The model under review builds one solid part; all positions refer to its coordinate system, in mm. Give positions to 0.01 mm unless a question says otherwise; leave off trailing zeros. Loops run counter-clockwise (first coordinate to the right, second up) from the corner with the lowest first, then second, coordinate; pieces in that order, holes last. Notation, with made-up numbers: M 25,63 L 46,63 A28 ccw 46,81 Z; hole C 15.5,25 d2. An arc over 180 degrees is marked long. Return JSON: item names as keys, results as strings. Group by question number.
```python
from build123d import *

# Parameters (mm, degrees)
SKETCH_1_W      = 220
SKETCH_1_H      = 54
SKETCH_1_R      = 2.1
SKETCH_1_R_2    = 2
SKETCH_1_R_3    = 14.5
EXTRUDE_1_DEPTH = 3
CHAMFER_1_SIZE  = 4


with BuildPart() as part:
    # 草图1 → 凸台-拉伸1 (new, symmetric)
    with BuildSketch(Plane.XY):
        Rectangle(SKETCH_1_W, SKETCH_1_H)
        with Locations((-100, 17)):
            Circle(SKETCH_1_R, mode=Mode.SUBTRACT)
        with Locations((-100, -17)):
            Circle(SKETCH_1_R, mode=Mode.SUBTRACT)
        with Locations((100, 17)):
            Circle(SKETCH_1_R, mode=Mode.SUBTRACT)
        with Locations((100, -17)):
            Circle(SKETCH_1_R, mode=Mode.SUBTRACT)
        with Locations((0, 17.5)):
            Circle(SKETCH_1_R_2, mode=Mode.SUBTRACT)
        Circle(SKETCH_1_R_3, mode=Mode.SUBTRACT)
        with Locations((17.5, 0)):
            Circle(SKETCH_1_R_2, mode=Mode.SUBTRACT)
        with Locations((0, -17.5)):
            Circle(SKETCH_1_R_2, mode=Mode.SUBTRACT)
        with Locations((-17.5, 0)):
            Circle(SKETCH_1_R_2, mode=Mode.SUBTRACT)
    extrude(amount=EXTRUDE_1_DEPTH, both=True)

    # 倒角1
    chamfer_1_edges = [part.edges().sort_by_distance(p)[0] for p in [
        (-110, 27, 0),
        (110, 27, 0),
        (110, -27, 0),
        (-110, -27, 0),
    ]]
    chamfer(chamfer_1_edges, length=CHAMFER_1_SIZE)


solid = part.part
```
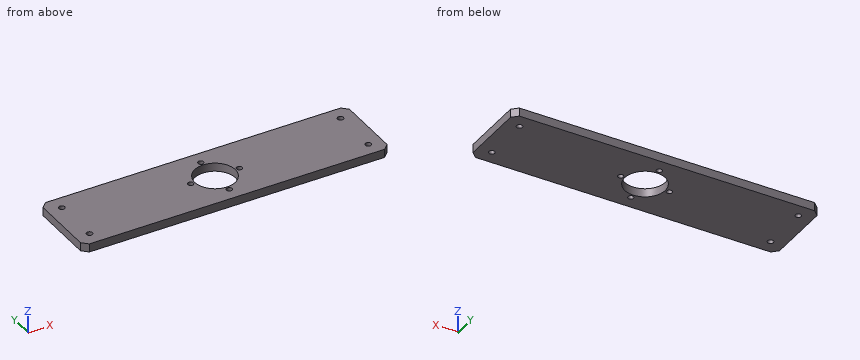
(1) For probe 1 along Y at (x, z) = (0, -1.7); probe 2 along Y at (x, z) = (100, 0.9); probe 3 along Y at (x, z) = (17.5, 0), list the stretches that pass through material, from the lowest coordinate up.
(2) Add section B-B (x = -100). Write out the cut boundary in (y, z), and give its area (3 significant figures).
(3) Add section C-C (y = -10). Write out the cut boundary in (x, z), and give its area (3 significant figures).
(4) Add section D-D (x = 6). Write out the cut boundary in (y, z).
(5) For pin 1 (6.5 mm diameter, centred on x = 17.5, y = 0, fed in from -Z), flat-tipped, find the tip position at first contact; note if it passes through.
(6) Add section A-A (z = 1.25). Count the separate pieces of the cut face and the enclosed holes in it, and give its area (3 significant figures).
Verdict:
{
 "1": {"probe 1": "y = -27 to -19.5, -15.5 to -14.5, 14.5 to 15.5, 19.5 to 27", "probe 2": "y = -27 to -19.1, -14.9 to 14.9, 19.1 to 27", "probe 3": "y = -27 to -2, 2 to 27"},
 "2": {"outline": "M -27,-3 L -19.1,-3 L -19.1,3 L -27,3 Z; M -14.9,-3 L 14.9,-3 L 14.9,3 L -14.9,3 Z; M 19.1,-3 L 27,-3 L 27,3 L 19.1,3 Z", "area": "274 mm²"},
 "3": {"outline": "M -110,-3 L -10.5,-3 L -10.5,3 L -110,3 Z; M 10.5,-3 L 110,-3 L 110,3 L 10.5,3 Z", "area": "1,190 mm²"},
 "4": {"outline": "M -27,-3 L -13.2,-3 L -13.2,3 L -27,3 Z; M 13.2,-3 L 27,-3 L 27,3 L 13.2,3 Z"},
 "5": {"pin 1": "stops at z = -3"},
 "6": {"separate pieces": "1", "enclosed holes": "9", "area": "11,100 mm²"}
}
